Geometry check sheet. Reference: the model listing, model coordinates, mm. Give positions to 0.01 mm unless a question says otherwise; leave off trailing zeros. Loops run counter-clockwise (first coordinate to the right, second up) from the corner with the lowest first, then second, coordinate; pieces in that order, holes last. Notation, with made-up numbers: (-2, 87) -> (50, 87) arc R17 cw to (50, 103) -> close; hole circle Ø10 at (48.5, 64). An arc over 180 degrees is marked (long way). Answer as a JSON object with one key per item and string values.
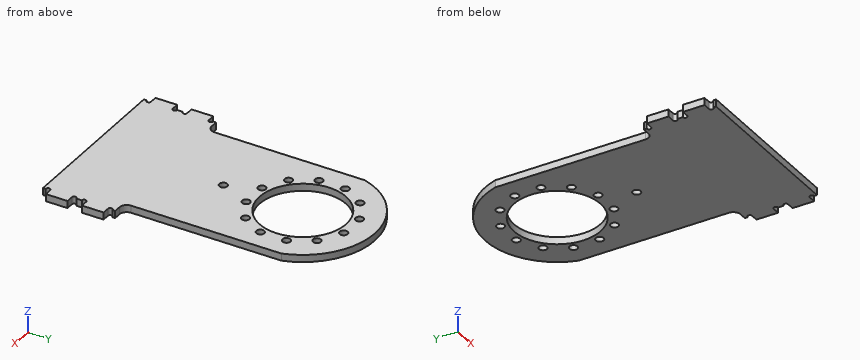
from build123d import *

# Parameters (mm, degrees)
SKETCH_1_R          = 30
EXTRUDE_1_DEPTH     = 5
SKETCH_3_R          = 2.75
CUT_EXTRUDE_2_DEPTH = 20
SKETCH_4_R          = 2.75
CUT_EXTRUDE_3_DEPTH = 10
SKETCH_5_W          = 116
SKETCH_5_H          = 50
EXTRUDE_2_DEPTH     = 5
SKETCH_8_W          = 5
SKETCH_8_H          = 15
EXTRUDE_3_DEPTH     = 5
SKETCH_9_R          = 1.55
CUT_EXTRUDE_6_DEPTH = 5
FILLET_1_R          = 5


with BuildPart() as part:
    # 草图1 → 凸台-拉伸1 (new body)
    with BuildSketch(Plane.XY):
        with BuildLine():
            Line((-48, 109.07), (-48, 0))
            Line((-48, 0), (48, 0))
            Line((48, 0), (48, 109.07))
            ThreePointArc((48, 109.07), (0, 145.07), (-48, 109.07))
        make_face()
        with Locations((0, 95.07)):
            Circle(SKETCH_1_R, mode=Mode.SUBTRACT)
    extrude(amount=EXTRUDE_1_DEPTH)

    # 草图3 → 切除-拉伸2 (cut)
    with BuildSketch(Plane.XY.offset(5)):
        with Locations((0, 40)):
            Circle(SKETCH_3_R)
    extrude(amount=-CUT_EXTRUDE_2_DEPTH, mode=Mode.SUBTRACT)

    # 草图4 → 切除-拉伸3 (cut)
    with BuildSketch(Plane.XY.offset(5)):
        with Locations((9.058666579, 128.87740392)):
            Circle(SKETCH_4_R)
        with Locations((24.748737342, 119.818737342)):
            Circle(SKETCH_4_R)
        with Locations((33.80740392, 104.128666579)):
            Circle(SKETCH_4_R)
        with Locations((33.80740392, 86.011333421)):
            Circle(SKETCH_4_R)
        with Locations((24.748737342, 70.321262658)):
            Circle(SKETCH_4_R)
        with Locations((9.058666579, 61.26259608)):
            Circle(SKETCH_4_R)
        with Locations((-9.058666579, 61.26259608)):
            Circle(SKETCH_4_R)
        with Locations((-24.748737342, 70.321262658)):
            Circle(SKETCH_4_R)
        with Locations((-33.80740392, 86.011333421)):
            Circle(SKETCH_4_R)
        with Locations((-33.80740392, 104.128666579)):
            Circle(SKETCH_4_R)
        with Locations((-24.748737342, 119.818737342)):
            Circle(SKETCH_4_R)
        with Locations((-9.058666579, 128.87740392)):
            Circle(SKETCH_4_R)
    extrude(amount=-CUT_EXTRUDE_3_DEPTH, mode=Mode.SUBTRACT)

    # 草图5 → 凸台-拉伸2 (add)
    with BuildSketch(Plane.XY.offset(5)):
        with Locations((0, -25)):
            Rectangle(SKETCH_5_W, SKETCH_5_H)
    extrude(amount=-EXTRUDE_2_DEPTH)

    # 草图8 → 凸台-拉伸3 (add)
    with BuildSketch(Plane.XY.offset(5)):
        with Locations((60.5, -12.5)):
            Rectangle(SKETCH_8_W, SKETCH_8_H)
        with Locations((60.5, -37.5)):
            Rectangle(SKETCH_8_W, SKETCH_8_H)
        with Locations((-60.5, -37.5)):
            Rectangle(SKETCH_8_W, SKETCH_8_H)
        with Locations((-60.5, -12.5)):
            Rectangle(SKETCH_8_W, SKETCH_8_H)
    extrude(amount=-EXTRUDE_3_DEPTH)

    # 草图9 → 切除-拉伸6 (cut)
    with BuildSketch(Plane.XY.offset(5)):
        with Locations((58, -3.45)):
            Circle(SKETCH_9_R)
        with Locations((58, -21.55)):
            Circle(SKETCH_9_R)
        with Locations((58, -28.45)):
            Circle(SKETCH_9_R)
        with Locations((58, -46.55)):
            Circle(SKETCH_9_R)
        with Locations((-58, -46.55)):
            Circle(SKETCH_9_R)
        with Locations((-58, -28.45)):
            Circle(SKETCH_9_R)
        with Locations((-58, -21.55)):
            Circle(SKETCH_9_R)
        with Locations((-58, -3.45)):
            Circle(SKETCH_9_R)
    extrude(amount=-CUT_EXTRUDE_6_DEPTH, mode=Mode.SUBTRACT)

    # 圆角1
    fillet_1_edges = [part.edges().sort_by_distance(p)[0] for p in [
        (48, 0, 2.5),
        (-48, 0, 2.5),
    ]]
    fillet(fillet_1_edges, radius=FILLET_1_R)


solid = part.part
1) Section check A-A on y = 40. Record the cut outline in (x, z), plus the area to 4 significant figures.
Geometry check:
{"outline": "(-48, 0) -> (-2.75, 0) -> (-2.75, 5) -> (-48, 5) -> close; (2.75, 0) -> (48, 0) -> (48, 5) -> (2.75, 5) -> close", "area": "452.5 mm2"}
2) Material ranges on line 1 along Y through (x, z) = (0, 1); line 2 along X through (y, z) = (117.5, 3.4); line 3 along X through (y, z) = (102.5, 1.8), recorded low to high. Write a range as from..to.
Geometry check:
{"line 1": "y = -50..37.25, 42.75..65.07, 125.07..145.07", "line 2": "x = -44.69..-26.23, -23.27..-19.92, 19.92..23.27, 26.23..44.69", "line 3": "x = -48..-36.02, -31.59..-29.07, 29.07..31.59, 36.02..48"}
3) Section check B-B on x = -24. Record the cut outline in (y, z), plus the area to 3 significant figures.
Geometry check:
{"outline": "(-50, 0) -> (67.68, 0) -> (67.68, 5) -> (-50, 5) -> close; (72.97, 0) -> (77.07, 0) -> (77.07, 5) -> (72.97, 5) -> close; (113.07, 0) -> (117.17, 0) -> (117.17, 5) -> (113.07, 5) -> close; (122.46, 0) -> (138.93, 0) -> (138.93, 5) -> (122.46, 5) -> close", "area": "712 mm2"}
4) Section check D-D on x = 17. Record the cut outline in (y, z), plus the area to 3 significant figures.
Geometry check:
{"outline": "(-50, 0) -> (70.35, 0) -> (70.35, 5) -> (-50, 5) -> close; (119.79, 0) -> (142.09, 0) -> (142.09, 5) -> (119.79, 5) -> close", "area": "713 mm2"}
5) Depth check by flat-ended pin: P1, Ø1.9, axis at y = -24.5, z = 1.5, coming from the -X side; P2, Ø0.6, axis at y = -0.5, z = 1.5, coming from the +X side; P3, Ø3.5, axis at x = -24.75, y = 70.32, coming from the +Z side; P4, Ø3, axis at y = 36, z = 0.5, coming from the -X side. Enter the tip coordinate at first touch or a pass-through.
Geometry check:
{"P1": "stops at x = -58", "P2": "stops at x = 58", "P3": "passes through", "P4": "stops at x = -48"}
6) Section check C-C on x = 0. Record the cut outline in (y, z).
Geometry check:
{"outline": "(-50, 0) -> (37.25, 0) -> (37.25, 5) -> (-50, 5) -> close; (42.75, 0) -> (65.07, 0) -> (65.07, 5) -> (42.75, 5) -> close; (125.07, 0) -> (145.07, 0) -> (145.07, 5) -> (125.07, 5) -> close"}
